from build123d import *

# Parameters (mm, degrees)
F1_DEPTH = 2


with BuildPart() as f1:
    # F0 (on Front) → F1 (new body, symmetric)
    with BuildSketch(Plane.XZ):
        with BuildLine():
            Line((12.124539, 2.9972), (0, 2.9972))
            Line((0, 2.9972), (-12.124539, 2.9972))
            ThreePointArc((-12.124539, 2.9972), (-17.406568, 4.032223), (-21.907339, 6.984201))
            ThreePointArc((-21.907339, 6.984201), (-26.785135, 10.083517), (-32.4993, 10.947792))
            Line((-32.4993, 10.947792), (-57.5056, 9.4996))
            Line((-57.5056, 9.4996), (-57.5056, 0))
            Line((-57.5056, 0), (-57.5056, -9.4996))
            Line((-57.5056, -9.4996), (-32.4993, -10.947792))
            ThreePointArc((-32.4993, -10.947792), (-26.785135, -10.083517), (-21.907339, -6.984201))
            ThreePointArc((-21.907339, -6.984201), (-17.406568, -4.032223), (-12.124539, -2.9972))
            Line((-12.124539, -2.9972), (0, -2.9972))
            Line((0, -2.9972), (12.124539, -2.9972))
            ThreePointArc((12.124539, -2.9972), (17.406568, -4.032223), (21.907339, -6.984201))
            ThreePointArc((21.907339, -6.984201), (26.785135, -10.083517), (32.4993, -10.947792))
            Line((32.4993, -10.947792), (57.5056, -9.4996))
            Line((57.5056, -9.4996), (57.5056, 0))
            Line((57.5056, 0), (57.5056, 9.4996))
            Line((57.5056, 9.4996), (32.4993, 10.947792))
            ThreePointArc((32.4993, 10.947792), (26.785135, 10.083517), (21.907339, 6.984201))
            ThreePointArc((21.907339, 6.984201), (17.406568, 4.032223), (12.124539, 2.9972))
        make_face()
    extrude(amount=F1_DEPTH, both=True)


solid = f1.part
The model under review builds one solid part; all positions refer to its coordinate system, in mm. A direction names the side the tool comes from. Coordinates: 2 decimals unless noted, no trailing zeros. Loops run counter-clockwise (first coordinate to the right, second up) from the corner with the lowest first, then second, coordinate; pieces in that order, holes last. Notation, with made-up numbers: (50, 17) -> (77, 17) arc R28 cw to (77, 37) -> close; hole circle Ø2 at (-30, -28). An arc over 180 degrees is marked (long way). Use a Markdown table: item, result. Add a question column.
1. To check wall thickness, follow line 1 (Z direction, x = 3.5, y = 1.7); line 2 (X direction, y = 0.5, z = -7.5); line 3 (X direction, y = -1.25, z = 6.5). State the ranges of each line that lie inside material, in increasing order.
2. Draft analysis for pull direction X (two halves, no side actions). For faces 1 (the face through (-17.336, -0.028, 4.004)), 2 (the face through (-26.86, -0.03, -10.11)), 3 (the face through (45.177, -0.028, 10.214)), 4 (the face through (-1, 2, 0)), state which applies: pulls with the +X half, pulls with the -X half, needs draft (parallel to the pull), parting line crosses it, or undercut.
3. Add section B-B on z = 5.25. Write out the cut boundary in (x, y).
4. Clearance check with flat-ended pins moving along their axes: pin 1 Ø8 at (x, z) = (-12, 7.5) entering from -Y; pin 2 Ø1.2 at (x, y) = (5, 0) entering from -Z. State where each tip first meets the part, or that it passes through.
5. Add section D-D on x = -47. Write out the cut boundary in (y, z), plus the area to 3 significant figures.
6. Add section A-A on y = -0.9. Write out the cut boundary in (x, z).
7. Machinability: for faces 5 (the face through (-17.477, -0.028, -4.061)), 6 (the face through (17.477, -0.028, 4.061)), 7 (the face through (-1, -2, 0)), which of the approach directions +Z, -Z, +X, -X, +Y, -Y give a long, thin tool a straight path to every point of the face, cutting with its end or side? Answer none if there is none.
8. Add section C-C on x = -5. Write out the cut boundary in (y, z), plus the area to 3 significant figures.
Returned:
| question | item | result |
|---|---|---|
| 1 | line 1 | z = -3 to 3 |
| 1 | line 2 | x = -57.51 to -22.46, 22.46 to 57.51 |
| 1 | line 3 | x = -57.51 to -21.39, 21.39 to 57.51 |
| 2 | face 1 | undercut |
| 2 | face 2 | undercut |
| 2 | face 3 | pulls with the +X half |
| 2 | face 4 | needs draft |
| 3 | outline | (-57.51, -2) -> (-19.74, -2) -> (-19.74, 2) -> (-57.51, 2) -> close; (19.74, -2) -> (57.51, -2) -> (57.51, 2) -> (19.74, 2) -> close |
| 4 | pin 1 | passes through |
| 4 | pin 2 | stops at z = -3 |
| 5 | outline | (-2, -10.11) -> (2, -10.11) -> (2, 10.11) -> (-2, 10.11) -> close |
| 5 | area | 80.9 mm² |
| 6 | outline | (-57.51, -9.5) -> (-32.5, -10.95) arc R14 ccw to (-21.91, -6.98) arc R14 cw to (-12.12, -3) -> (12.12, -3) arc R14 cw to (21.91, -6.98) arc R14 ccw to (32.5, -10.95) -> (57.51, -9.5) -> (57.51, 9.5) -> (32.5, 10.95) arc R14 ccw to (21.91, 6.98) arc R14 cw to (12.12, 3) -> (-12.12, 3) arc R14 cw to (-21.91, 6.98) arc R14 ccw to (-32.5, 10.95) -> (-57.51, 9.5) -> close |
| 7 | face 5 | -Z, +Y, -Y |
| 7 | face 6 | +Z, +Y, -Y |
| 7 | face 7 | +Z, -Z, +X, -X, -Y |
| 8 | outline | (-2, -3) -> (2, -3) -> (2, 3) -> (-2, 3) -> close |
| 8 | area | 24.0 mm² |
